Geometry: final body of the model. Coordinates: model frame, mm. Face numbers are marked on the shaded views. A direction names the side the tool comes from. Round coordinates to 2 decimals unless told otherwise and drop trailing zeros. Order: outer loops, then holes, each group sorted by start corner. A loop starts at its lowest first (then second) coordinate and runs counter-clockwise, first axis right, second up. Notation, with made-up numbers: M 48,78.25 L 76,78.25 A23 cw 76,98.25 Z; hole C 72,22 d2. An arc over 180 degrees is marked long. Return JSON: item names as keys, results as strings. Group by question number.
Q1. Cut plane C-C on z = -1.5. Output: boundary loops of the cut face in (x, y).
Q2. Ray query, probe 1 along Z at (x, y) = (14, 26); probe 2 along Z at (x, y) = (-1, 6.5); probe 3 along X at (y, z) = (50, -1). Return the intervals inside material, ascending.
Q3. Cut plane B-B on x = 0. Output: boundary loops of the cut face in (y, z).
Q4. Contact query for flat-ended pins moving along their axis: pin 1 (5 mm diameter, centred on x = 13, y = 30, fed in from +Z); pin 2 (1.5 mm diameter, centred on x = 1.5, y = 23.5, fed in from -Z); pin 3 (1.5 mm diameter, centred on x = 3, y = 43, fed in from +Z). Output: stop coordinate, or through.
Q5. Cut plane A-A on y = 15. Output: boundary loops of the cut face in (x, z).
Q6. Access query for the marked faces 1, 2 and 3. Directions: +Z, -Z, +X, -X, +Y, -Y. A direction counts if a zero-diameter tool reaches every point of the face in a straight line with its end or side. Return the directions, or none.
Q7. Cut plane D-D on y = 46. Output: boundary loops of the cut face in (x, z), and give its area (3 significant figures).
```python
from build123d import *

# Parameters (mm, degrees)
SKETCH_1_R          = 2.5
EXTRUDE_1_DEPTH     = 30
CUT_EXTRUDE_1_REACH = 37.984
SKETCH_2_R          = 2
FILLET_1_R          = 1
SKETCH_3_R          = 2.5
EXTRUDE_2_DEPTH     = 60.5
SKETCH_4_R          = 3.55
EXTRUDE_3_DEPTH     = 1
SKETCH_5_R          = 3.55
SKETCH_5_R_2        = 2.5
EXTRUDE_4_DEPTH     = 0.5


with BuildPart() as part:
    # 草图1 → 凸台-拉伸1 (new body)
    with BuildSketch(Plane(origin=(0, 0, 0), x_dir=(1, 0, 0), z_dir=(0, 1, 0))):
        with BuildLine():
            Line((19.464101615, -0.5), (3.464101615, -0.5))
            ThreePointArc((3.464101615, -0.5), (-3.5, 0), (3.464101615, 0.5))
            Line((3.464101615, 0.5), (19.464101615, 0.5))
            Line((19.464101615, 0.5), (19.464101615, -0.5))
        make_face()
        with Locations(Location((0, 0, 0), (0, 0, 270))):
            Circle(SKETCH_1_R, mode=Mode.SUBTRACT)
    extrude(amount=EXTRUDE_1_DEPTH)

    # 草图2 → 切除-拉伸1 (cut, up to next)
    with BuildSketch(Plane.XY.offset(0.5), mode=Mode.PRIVATE) as cut_extrude_1_sk1:
        with Locations((14.464101615, 24)):
            Circle(SKETCH_2_R)
    cut_extrude_1_tool1 = extrude(cut_extrude_1_sk1.sketch, amount=-CUT_EXTRUDE_1_REACH, mode=Mode.PRIVATE) & part.part
    # 草图2 → 切除-拉伸1 (cut, up to next)
    with BuildSketch(Plane.XY.offset(0.5), mode=Mode.PRIVATE) as cut_extrude_1_sk2:
        with Locations((8.139546295, 15)):
            Circle(SKETCH_2_R)
    cut_extrude_1_tool2 = extrude(cut_extrude_1_sk2.sketch, amount=-CUT_EXTRUDE_1_REACH, mode=Mode.PRIVATE) & part.part
    # 草图2 → 切除-拉伸1 (cut, up to next)
    with BuildSketch(Plane.XY.offset(0.5), mode=Mode.PRIVATE) as cut_extrude_1_sk3:
        with Locations((14.464101615, 6)):
            Circle(SKETCH_2_R)
    cut_extrude_1_tool3 = extrude(cut_extrude_1_sk3.sketch, amount=-CUT_EXTRUDE_1_REACH, mode=Mode.PRIVATE) & part.part
    add(cut_extrude_1_tool1.solids().sort_by_distance((14.464102, 24, 0.5))[0], mode=Mode.SUBTRACT)
    add(cut_extrude_1_tool2.solids().sort_by_distance((8.139546, 15, 0.5))[0], mode=Mode.SUBTRACT)
    add(cut_extrude_1_tool3.solids().sort_by_distance((14.464102, 6, 0.5))[0], mode=Mode.SUBTRACT)

    # 圆角1
    fillet_1_edges = [part.edges().sort_by_distance(p)[0] for p in [
        (19.464101615, 30, 0),
        (19.464101615, 0, 0),
    ]]
    fillet(fillet_1_edges, radius=FILLET_1_R)

    # 草图3 → 凸台-拉伸2 (add)
    with BuildSketch(Plane.XZ):
        with Locations(Location((0, 0, 0), (0, 0, 270))):
            Circle(SKETCH_3_R)
    extrude(amount=-EXTRUDE_2_DEPTH)

    # 草图4 → 凸台-拉伸3 (add)
    with BuildSketch(Plane.XZ):
        with Locations(Location((0, 0, 0), (0, 0, 8.09674977))):
            Circle(SKETCH_4_R)
    extrude(amount=EXTRUDE_3_DEPTH)

    # 草图5 → 凸台-拉伸4 (add)
    with BuildSketch(Plane(origin=(0, 30, 0), x_dir=(1, 0, 0), z_dir=(0, 1, 0))):
        with Locations(Location((0, 0, 0), (0, 0, 351.90325023))):
            Circle(SKETCH_5_R)
        with Locations(Location((0, 0, 0), (0, 0, 90))):
            Circle(SKETCH_5_R_2, mode=Mode.SUBTRACT)
    extrude(amount=EXTRUDE_4_DEPTH)


solid = part.part
```
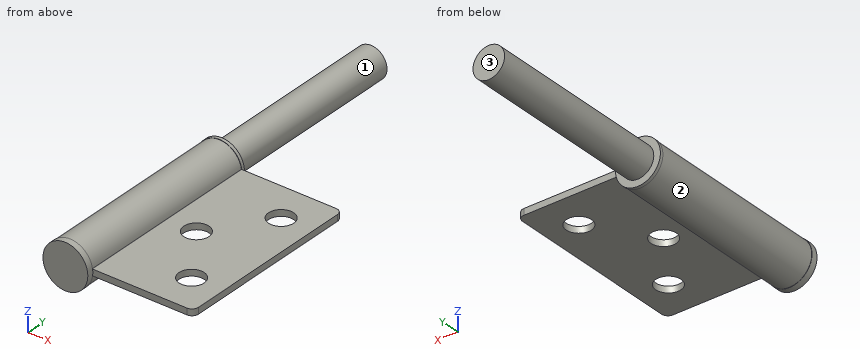
Result sheet:
{
 "1": {"outline": "M -3.22,-1 L 3.22,-1 L 3.22,0 L 3.16,0 L 3.16,30 L 3.22,30 L 3.22,30.5 L 2,30.5 L 2,60.5 L -2,60.5 L -2,30.5 L -3.22,30.5 L -3.22,30 L -3.16,30 L -3.16,0 L -3.22,0 Z"},
 "2": {"probe 1": "z = -0.5 to 0.5", "probe 2": "z = -3.35 to 3.35", "probe 3": "x = -2.29 to 2.29"},
 "3": {"outline": "M -1,-3.55 L 0,-3.55 L 0,-3.5 L 30,-3.5 L 30,-3.55 L 30.5,-3.55 L 30.5,-2.5 L 60.5,-2.5 L 60.5,2.5 L 30.5,2.5 L 30.5,3.55 L 30,3.55 L 30,3.5 L 0,3.5 L 0,3.55 L -1,3.55 Z"},
 "4": {"pin 1": "stops at z = 0.5", "pin 2": "stops at z = -3.42", "pin 3": "stops at z = 1.09"},
 "5": {"outline": "M 3.46,-0.5 L 6.14,-0.5 L 6.14,0.5 L 3.46,0.5 A3.5 ccw long Z; M 10.14,-0.5 L 19.46,-0.5 L 19.46,0.5 L 10.14,0.5 Z"},
 "6": {"face 1": "+Y", "face 2": "none", "face 3": "+Z, -Z, +X, -X, +Y"},
 "7": {"outline": "C 0,0 d5", "area": "19.6 mm²"}
}
